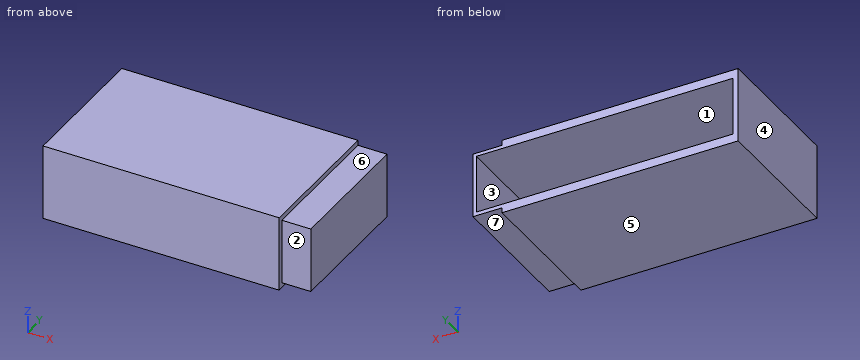
```python
from build123d import *

# Parameters (mm, degrees)
SKETCH5_W           = 317.643030656
SKETCH5_H           = 101.565982789
BOSS_EXTRUDE3_DEPTH = 190.5
SKETCH11_W          = 310.281709158
SKETCH11_H          = 87.664375102
CUT_EXTRUDE2_DEPTH  = 184.15
SKETCH14_W          = 87.664375102
SKETCH14_H          = 184.15
BOSS_EXTRUDE5_DEPTH = 349.25
SKETCH18_W          = 345.261683736
SKETCH18_H          = 78.300417561
CUT_EXTRUDE3_DEPTH  = 181.61


with BuildPart() as part:
    # Sketch5 → Boss-Extrude3 (new body)
    with BuildSketch(Plane(origin=(0, 0, 0), x_dir=(1, 0, 0), z_dir=(0, 1, 0))):
        with Locations((-31.847605324, 64.703654394)):
            Rectangle(SKETCH5_W, SKETCH5_H)
    extrude(amount=BOSS_EXTRUDE3_DEPTH)

    # Sketch11 → Cut-Extrude2 (cut)
    with BuildSketch(Plane(origin=(0, 190.5, 0), x_dir=(1, 0, 0), z_dir=(0, 1, 0))):
        with Locations((-28.166944575, 64.789017072)):
            Rectangle(SKETCH11_W, SKETCH11_H)
    extrude(amount=-CUT_EXTRUDE2_DEPTH, mode=Mode.SUBTRACT)

    # Sketch14 → Boss-Extrude5 (add)
    with BuildSketch(Plane(origin=(-183.307799154, 0, 0), x_dir=(0, 0, -1), z_dir=(1, 0, 0))):
        with Locations((64.789017072, 98.425)):
            Rectangle(SKETCH14_W, SKETCH14_H)
    extrude(amount=BOSS_EXTRUDE5_DEPTH)

    # Sketch18 → Cut-Extrude3 (cut)
    with BuildSketch(Plane(origin=(0, 190.5, 0), x_dir=(1, 0, 0), z_dir=(0, 1, 0))):
        with Locations((-11.130382461, 64.549519714)):
            Rectangle(SKETCH18_W, SKETCH18_H)
    extrude(amount=-CUT_EXTRUDE3_DEPTH, mode=Mode.SUBTRACT)


solid = part.part
```
Can you work these out from the model? Positions are in its coordinate system, mm. Face numbers are marked on the shaded views. A direction names the side the tool comes from. Coordinates: 2 decimals unless noted, no trailing zeros. Write each loop counter-clockwise with the first axis right and the second up, starting at its lowest first coordinate (ties: lowest second). Pieces come first, ordered by that corner, then holes. Notation, with made-up numbers: M 47,-0.5 L 55,-0.5 A17 ccw 55,12.5 Z; hole C -30,-21 d1. An arc over 180 degrees is marked long. Answer as CSV lines item,"result".
Item 1: We'd pull the mould along X, two halves only. Please class the marked faces 1, 2, 3 and 4: +X half, -X half, draft (parallel to the pull), parting line (faces both ways), or undercut.
Geometry results:
face 1,"undercut"
face 2,"draft"
face 3,"undercut"
face 4,"-X half"
Item 2: Please list where these lines run through material, in increasing order: line 1 along Z through (x, y) = (-93, 109.5); line 2 along X through (y, z) = (144, -40); line 3 along Z through (x, y) = (148, 99).
Geometry results:
line 1,"z = -115.49 to -103.7, -25.4 to -13.92"
line 2,"x = -190.67 to -183.76, 161.5 to 165.94"
line 3,"z = -108.62 to -103.7, -25.4 to -20.96"
Item 3: Imagine slicing it at C-C on x = 131. List the corners of the cut face in (y, z) for me.
Geometry results:
outline,"M 6.35,-108.62 L 190.5,-108.62 L 190.5,-103.7 L 8.89,-103.7 L 8.89,-25.4 L 190.5,-25.4 L 190.5,-20.96 L 6.35,-20.96 Z"
Item 4: On a 3-axis mill with a long thin cutter (end or side, diameter ignored), from which of +Z, -Z, +X, -X, +Y, -Y can I reach the whole of each face in a straight line? I mean the marked faces 5, 6 and 7. Say none if no direction works.
Geometry results:
face 5,"-Z, +X, -X, +Y, -Y"
face 6,"+Z, +X, +Y, -Y"
face 7,"-Z, +X, +Y, -Y"
Item 5: I'm going to push flat-ended pins straight in: P1, Ø23.5, axis at x = -9, z = -50.5, coming from the +Y side; P2, Ø19.5, axis at x = 148.5, y = 77, coming from the +Z side; P3, Ø19.5, axis at x = 153.5, y = 90, coming from the -Z side. Where does each tip first touch, or does it pass through?
Geometry results:
P1,"stops at y = 8.89"
P2,"stops at z = -20.96"
P3,"stops at z = -108.62"
Item 6: Imagine slicing it at B-B on z = -76. List the corners of the cut face in (x, y) for me, plus the area to 3 significant figures.
Geometry results:
outline,"M -190.67,0 L 126.97,0 L 126.97,6.35 L 165.94,6.35 L 165.94,190.5 L 161.5,190.5 L 161.5,8.89 L -183.76,8.89 L -183.76,190.5 L -190.67,190.5 Z"
area,"4,980 mm2"
Item 7: Imagine slicing it at D-D on x = -141. List the corners of the cut face in (y, z) for me, plus the area to 3 significant figures.
Geometry results:
outline,"M 0,-115.49 L 190.5,-115.49 L 190.5,-103.7 L 8.89,-103.7 L 8.89,-25.4 L 190.5,-25.4 L 190.5,-13.92 L 0,-13.92 Z"
area,"5,130 mm2"
Item 8: Imagine slicing it at A-A on y = 16. List the corners of the cut face in (x, z) for me.
Geometry results:
outline,"M -190.67,-115.49 L 126.97,-115.49 L 126.97,-108.62 L 165.94,-108.62 L 165.94,-20.96 L 126.97,-20.96 L 126.97,-13.92 L -190.67,-13.92 Z; hole M -183.76,-103.7 L 161.5,-103.7 L 161.5,-25.4 L -183.76,-25.4 Z"
